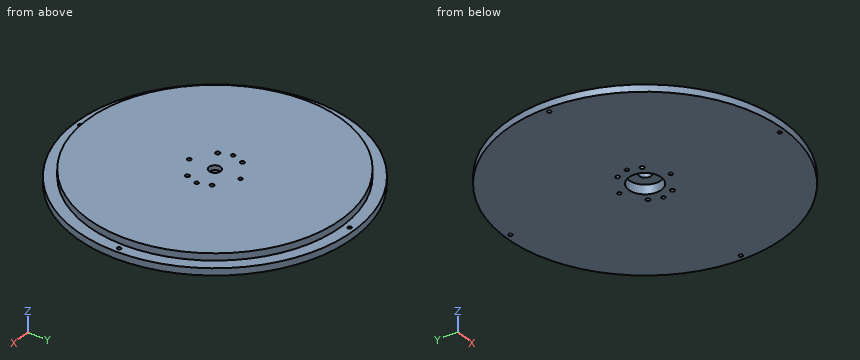
```python
from build123d import *

# Parameters (mm, degrees)
SKETCH_1_R          = 109.75
EXTRUDE_1_DEPTH     = 12
SKETCH_2_R          = 119.75
EXTRUDE_2_DEPTH     = 6
SKETCH_3_R          = 1.6
CUT_EXTRUDE_1_DEPTH = 10
SKETCH_4_R          = 1.6
CUT_EXTRUDE_2_DEPTH = 20
SKETCH_4_5_R        = 1.6
CUT_EXTRUDE_3_DEPTH = 20
SKETCH_6_R          = 5
CUT_EXTRUDE_5_DEPTH = 20
SKETCH_7_R          = 1.8
CUT_EXTRUDE_8_DEPTH = 30
SKETCH_10_R         = 14
CUT_EXTRUDE_9_DEPTH = 8


with BuildPart() as part:
    # 草图1 → 凸台-拉伸1 (new body)
    with BuildSketch(Plane.XY):
        Circle(SKETCH_1_R)
    extrude(amount=EXTRUDE_1_DEPTH)

    # 草图2 → 凸台-拉伸2 (add)
    with BuildSketch(Plane.XY):
        Circle(SKETCH_2_R)
    extrude(amount=EXTRUDE_2_DEPTH)

    # 草图3 → 切除-拉伸1 (cut)
    with BuildSketch(Plane.XY):
        with Locations((-115, 0)):
            Circle(SKETCH_3_R)
        with Locations((115, 0)):
            Circle(SKETCH_3_R)
        with Locations((0, -115)):
            Circle(SKETCH_3_R)
        with Locations((0, 115)):
            Circle(SKETCH_3_R)
    extrude(amount=CUT_EXTRUDE_1_DEPTH, mode=Mode.SUBTRACT)

    # 草图4 → 切除-拉伸2 (cut)
    with BuildSketch(Plane(origin=(0, 0, 0), x_dir=(-1, 0, 0), z_dir=(0, 0, -1))):
        with Locations((0, -21.9203)):
            Circle(SKETCH_4_R)
    extrude(amount=-CUT_EXTRUDE_2_DEPTH, mode=Mode.SUBTRACT)

    # 草图4<5> → 切除-拉伸3 (cut)
    with BuildSketch(Plane(origin=(0, 0, 0), x_dir=(-1, 0, 0), z_dir=(0, 0, -1))):
        with Locations((-21.9203, 0)):
            Circle(SKETCH_4_5_R)
        with Locations((0, 21.9203)):
            Circle(SKETCH_4_5_R)
        with Locations((21.9203, 0)):
            Circle(SKETCH_4_5_R)
        with Locations((0, -21.9203)):
            Circle(SKETCH_4_5_R)
    extrude(amount=-CUT_EXTRUDE_3_DEPTH, mode=Mode.SUBTRACT)

    # 草图6 → 切除-拉伸5 (cut)
    with BuildSketch(Plane(origin=(0, 0, 0), x_dir=(-1, 0, 0), z_dir=(0, 0, -1))):
        Circle(SKETCH_6_R)
    extrude(amount=-CUT_EXTRUDE_5_DEPTH, mode=Mode.SUBTRACT)

    # 草图7 → 切除-拉伸8 (cut)
    with BuildSketch(Plane(origin=(0, 0, 0), x_dir=(-1, 0, 0), z_dir=(0, 0, -1))):
        with Locations((-18.186533479, 10.5)):
            Circle(SKETCH_7_R)
        with Locations((18.186533479, 10.5)):
            Circle(SKETCH_7_R)
        with Locations((18.186533479, -10.5)):
            Circle(SKETCH_7_R)
        with Locations((-18.186533479, -10.5)):
            Circle(SKETCH_7_R)
    extrude(amount=-CUT_EXTRUDE_8_DEPTH, mode=Mode.SUBTRACT)

    # 草图10 → 切除-拉伸9 (cut)
    with BuildSketch(Plane(origin=(0, 0, 0), x_dir=(-1, 0, 0), z_dir=(0, 0, -1))):
        Circle(SKETCH_10_R)
    extrude(amount=-CUT_EXTRUDE_9_DEPTH, mode=Mode.SUBTRACT)


solid = part.part
```
For this review, take the finished solid that the model builds, in its own axes (mm). Coordinates: 2 decimals unless noted, no trailing zeros. Write each loop counter-clockwise with the first axis right and the second up, starting at its lowest first coordinate (ties: lowest second). Pieces come first, ordered by that corner, then holes.
(1) For pin 1 Ø2 at (x, y) = (18.19, 10.5) entering from +Z; pin 2 Ø5 at (y, z) = (35.5, 6) entering from +X; pin 3 Ø2 at (x, z) = (36, 4.5) entering from +Y; pin 4 Ø1 at (y, z) = (92.5, 8) entering from +X, all flat-tipped, find the tip position at first contact; note any pin that passes through.
(2) Add section B-B on z = 10. Count the separate pieces of the cut face and the enclosed holes in it, then the cut area to 3 significant figures.
(3) Wall thickness on probe 1 along Y at (x, z) = (0, 4); probe 2 along Y at (x, z) = (-27, 4); probe 3 along Z at (x, y) = (-103, -53): over which ranges is each line inside the solid? List them lowest first.
(4) Add section C-C on y = -83. Give the boundary of the cut face in (x, z), then the cut area to 3 significant figures.
(5) Add section A-A on x = -98.5. Give the boundary of the cut face in (y, z), then the cut area to 3 significant figures.
Answer sheet:
1. pin 1: passes through
1. pin 2: stops at x = 115.11
1. pin 3: stops at y = 114.52
1. pin 4: stops at x = 59.84
2. separate pieces: 1
2. enclosed holes: 9
2. area: 37,700 mm2
3. probe 1: y = -119.75 to -116.6, -113.4 to -23.52, -20.32 to -14, 14 to 20.32, 23.52 to 113.4, 116.6 to 119.75
3. probe 2: y = -116.67 to 116.67
3. probe 3: z = 0 to 6
4. outline: (-86.32, 0) - (86.32, 0) - (86.32, 6) - (71.81, 6) - (71.81, 12) - (-71.81, 12) - (-71.81, 6) - (-86.32, 6) - close
4. area: 1,900 mm2
5. outline: (-68.1, 0) - (68.1, 0) - (68.1, 6) - (48.4, 6) - (48.4, 12) - (-48.4, 12) - (-48.4, 6) - (-68.1, 6) - close
5. area: 1,400 mm2
